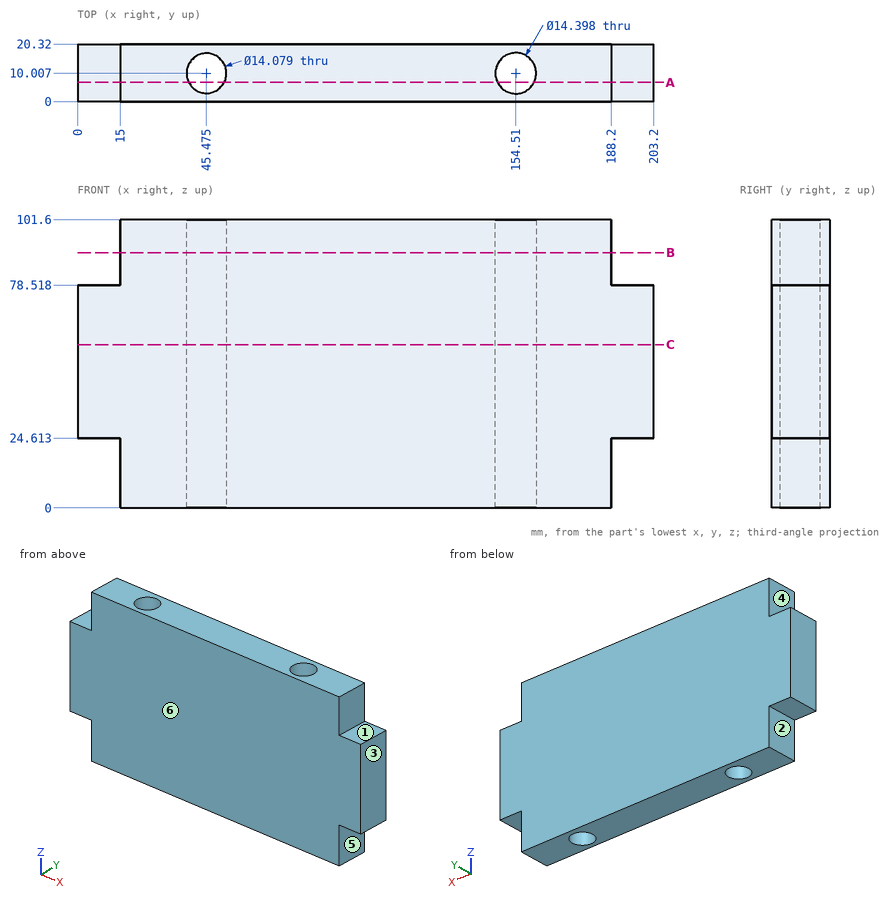
Could you check a few things on this drawing? It's one solid part, dimensions in mm from its lowest x, y, z. A direction names the side the tool comes from. Coordinates: 2 decimals unless noted, no trailing zeros. Loops run counter-clockwise (first coordinate to the right, second up) from the corner with the lowest first, then second, coordinate; pieces in that order, holes last.
1. For the marked faces 1, 2 and 3, which set-ups out of +Z, -Z, +X, -X, +Y, -Y let a thin tool reach every point of the face, with its end or its side?
2. Imagine slicing it at C-C (z = 57.5). Please give me the cut outline in (x, y) (1 decimal), and give its area (3 significant figures).
3. We'd pull the mould along X, two halves only. Please class the marked faces 4, 5 and 6: released by +X, released by -X, zero draft, split by the parting line, or undercut.
4. Imagine slicing it at B-B (z = 90). Please give me the cut outline in (x, y) (1 decimal), and give its area (3 significant figures).
5. Imagine slicing it at A-A (y = 6.75). Please give me the cut outline in (x, z) (1 decimal).
6. I need wall thicknesses on L1, parallel to X at y = 9.5, z = 33 (1 decimal); L2, parallel to X at y = 10, z = 74 (1 decimal); L3, parallel to X at y = 1, z = 8. Which ranges of each line are inside material? Lowest first, please.
7. For P1, Ø4.5, axis at x = 7.5, y = 7.5, coming from the +Z side; P2, Ø3, axis at y = 4.5, z = 15, coming from the -X side; P3, Ø6, axis at y = 12.5, z = 9, coming from the +X side, each with a flat end and sliding along its axis, tell me the tip position at first contact or that it passes through.
Computed values:
1. face 1: +Z, +X, +Y, -Y
1. face 2: -Z, -X, +Y, -Y
1. face 3: +Z, -Z, +X, +Y, -Y
2. outline: (0, 0) - (203.2, 0) - (203.2, 20.3) - (0, 20.3) - close; hole circle Ø14.1 at (45.5, 10); hole circle Ø14.4 at (154.5, 10)
2. area: 3,810 mm2
3. face 4: released by -X
3. face 5: released by +X
3. face 6: zero draft
4. outline: (15, 0) - (188.2, 0) - (188.2, 20.3) - (15, 20.3) - close; hole circle Ø14.1 at (45.5, 10); hole circle Ø14.4 at (154.5, 10)
4. area: 3,200 mm2
5. outline: (0, 24.6) - (15, 24.6) - (15, 0) - (39.2, 0) - (39.2, 101.6) - (15, 101.6) - (15, 78.5) - (0, 78.5) - close; (51.7, 0) - (148.1, 0) - (148.1, 101.6) - (51.7, 101.6) - close; (160.9, 0) - (188.2, 0) - (188.2, 24.6) - (203.2, 24.6) - (203.2, 78.5) - (188.2, 78.5) - (188.2, 101.6) - (160.9, 101.6) - close
6. L1: x = 0 to 38.5, 52.5 to 147.3, 161.7 to 203.2
6. L2: x = 0 to 38.4, 52.5 to 147.3, 161.7 to 203.2
6. L3: x = 15 to 188.2
7. P1: stops at z = 78.52
7. P2: stops at x = 15
7. P3: stops at x = 188.2
